from build123d import *

# Parameters (mm, degrees)
BOSS_EXTRUDE4_DEPTH = 50
SKETCH1_7_W         = 5
SKETCH1_7_H         = 15
SKETCH1_7_W_2       = 10
BOSS_EXTRUDE5_DEPTH = 60
SKETCH5_W           = 40
SKETCH5_H           = 33
CUT_EXTRUDE1_DEPTH  = 120
BOSS_EXTRUDE6_START = 15
BOSS_EXTRUDE6_DEPTH = 15
CUT_EXTRUDE3_DEPTH  = 67


with BuildPart() as part:
    # Sketch1 → Boss-Extrude4 (new, symmetric)
    with BuildSketch(Plane(origin=(0, 0, 0), x_dir=(1, 0, 0), z_dir=(0, 1, 0))):
        with BuildLine():
            Line((0, 0), (0, 15))
            Line((0, 15), (-20, 15))
            ThreePointArc((-20, 15), (-27.071067812, 17.928932188), (-30, 25))
            Line((-30, 25), (-30, 51))
            Line((-30, 51), (-40, 51))
            Line((-40, 51), (-40, 66))
            Line((-40, 66), (-30, 66))
            Line((-30, 66), (-30, 81))
            ThreePointArc((-30, 81), (-74.753734942, 32.115625929), (-40, -24.318022962))
            Line((-40, -24.318022962), (-40, 0))
            Line((-40, 0), (0, 0))
        make_face()
    extrude(amount=BOSS_EXTRUDE4_DEPTH, both=True)

    # Sketch1_7 → Boss-Extrude5 (add, symmetric)
    with BuildSketch(Plane(origin=(0, 0, 0), x_dir=(1, 0, 0), z_dir=(0, 1, 0))):
        with Locations((-27.5, 58.5)):
            Rectangle(SKETCH1_7_W, SKETCH1_7_H)
        with Locations((-35, 58.5)):
            Rectangle(SKETCH1_7_W_2, SKETCH1_7_H)
    extrude(amount=BOSS_EXTRUDE5_DEPTH, both=True)

    # Sketch5 → Cut-Extrude1 (cut)
    with BuildSketch(Plane(origin=(0, 0, 0), x_dir=(0, 0, -1), z_dir=(1, 0, 0))):
        with Locations((61, 3.5)):
            Rectangle(SKETCH5_W, SKETCH5_H)
    extrude(amount=-CUT_EXTRUDE1_DEPTH, mode=Mode.SUBTRACT)

    # Sketch6 → Boss-Extrude6 (add)
    with BuildSketch(Plane(origin=(0, 50, 0), x_dir=(1, 0, 0), z_dir=(0, 1, 0)).offset(BOSS_EXTRUDE6_START)):
        with BuildLine():
            Line((0, 5), (-74.666698166, 20.870896633))
            ThreePointArc((-74.666698166, 20.870896633), (-63.638154949, -6.560297565), (-40, -24.318022962))
            Line((-40, -24.318022962), (-40, 0))
            Line((-40, 0), (0, 0))
            Line((0, 0), (0, 5))
        make_face()
    extrude(amount=-BOSS_EXTRUDE6_DEPTH)

    # Sketch8 → Cut-Extrude3 (cut)
    with BuildSketch(Plane(origin=(0, 0, -15), x_dir=(-1, 0, 0), z_dir=(0, 0, -1))):
        with BuildLine():
            Line((15, 40), (15, -40))
            ThreePointArc((15, -40), (10, -45), (5, -40))
            Line((5, -40), (5, 40))
            ThreePointArc((5, 40), (10, 45), (15, 40))
        make_face()
    extrude(amount=-CUT_EXTRUDE3_DEPTH, mode=Mode.SUBTRACT)


solid = part.part
The model under review builds one solid part; all positions refer to its coordinate system, in mm. A direction names the side the tool comes from. Round coordinates to 2 decimals unless told otherwise and drop trailing zeros. Write each loop counter-clockwise with the first axis right and the second up, starting at its lowest first coordinate (ties: lowest second). Pieces come first, ordered by that corner, then holes. Notation, with made-up numbers: (-28, 86.25) -> (4, 86.25) arc R14 ccw to (4, 103.25) -> close; hole circle Ø2 at (-5.5, 51.25). An arc over 180 degrees is marked (long way). Answer as a JSON object with one key per item and string values.
1. Machinability: for faces 4 (the face through (-29, 45, -51)), 5 (the face through (-10, 45, -8)), 6 (the face through (-43, 20, -56)), 7 (the face through (-3, 1, -15)), 8 (the face through (-40, 8, 12)), which of the approach directions +Z, -Z, +X, -X, +Y, -Y give a long, thin tool a straight path to every point of the face, cutting with its end or side? Answer none if there is none.
Results found:
{"face 4": "+X, +Y", "face 5": "+Z, -Z", "face 6": "-Z, +X, -X", "face 7": "-Z, +X, +Y, -Y", "face 8": "+Z, +X, +Y, -Y"}
2. The part is to be moulded in two halves that separate along Y. For faces 1 (the face through (-25, 8, 0)), 2 (the face through (-10, -45, -8)), 3 (the face through (-33, 60, -59)), say which applies: pulls with the +Y half, pulls with the -Y half, needs draft (parallel to the pull), parting line crosses it, or undercut.
Results found:
{"face 1": "needs draft", "face 2": "undercut", "face 3": "pulls with the +Y half"}
3. We need section B-B on z = -11. State the section outline as (x, y) points.
Results found:
{"outline": "(-72.65, -50) -> (0, -50) -> (0, 50) -> (-28.23, 50) -> (-28.23, 65) -> (-72.65, 65) -> close; hole (-15, -40) arc R5 ccw to (-5, -40) -> (-5, 40) arc R5 ccw to (-15, 40) -> close"}
4. We need section D-D on x = -50. State the section outline as (y, z) points.
Results found:
{"outline": "(-50, -73.01) -> (-13, -73.01) -> (-13, -41) -> (20, -41) -> (20, -73.01) -> (50, -73.01) -> (50, -15.63) -> (65, -15.63) -> (65, 19.18) -> (-50, 19.18) -> close"}
5. We need section C-C on x = -10. State the section outline as (y, z) points, and give its area (3 significant figures).
Results found:
{"outline": "(-50, -15) -> (-45, -15) -> (-45, 0) -> (-50, 0) -> close; (45, -15) -> (50, -15) -> (50, -7.13) -> (65, -7.13) -> (65, 0) -> (45, 0) -> close", "area": "257 mm^2"}
6. Clearance check with flat-ended pins moving along their axes: pin 1 (4.5 mm diameter, centred on y = 9, z = -8, fed in from -X); pin 2 (3 mm diameter, centred on y = 54.5, z = -58, fed in from -X); pin 3 (12 mm diameter, centred on y = -25.5, z = -31, fed in from +X). State where each tip first meets the part, or that it passes through.
Results found:
{"pin 1": "stops at x = -72.41", "pin 2": "stops at x = -40", "pin 3": "stops at x = -30"}
7. To check wall thickness, follow line 1 along Y through (x, z) = (-49.5, -64); line 2 along Y through (x, z) = (-65, 3.5); line 3 along Y through (x, z) = (-68.5, -21). State the ranges of each line that lie inside material, in increasing order.
Results found:
{"line 1": "y = -50 to -13, 20 to 50", "line 2": "y = -50 to 65", "line 3": "y = -50 to 50"}
8. We need section A-A on y = 36. State the section outline as (x, z) points, and give its area (3 significant figures).
Results found:
{"outline": "(-40, 0) -> (-40, 24.32) arc R55 ccw to (-30, -81) -> (-30, -66) -> (-25, -66) -> (-25, -51) -> (-30, -51) -> (-30, -25) arc R10 cw to (-20, -15) -> (-15, -15) -> (-15, 0) -> close; (-5, -15) -> (0, -15) -> (0, 0) -> (-5, 0) -> close", "area": "3,800 mm^2"}
